Job drawing, mm, ordinate dimensions from the low corner. One solid piece. A direction names the side the tool comes from. Coordinates: 2 decimals unless noted, no trailing zeros. Loops run counter-clockwise (first coordinate to the right, second up) from the corner with the lowest first, then second, coordinate; pieces in that order, holes last. Notation, with made-up numbers: (53, 86) -> (107, 86) arc R17 cw to (107, 114) -> close; hole circle Ø3 at (-40, 22). An arc over 180 degrees is marked (long way). Use one line per item in the form item = value. Start each with the question number.
(1) Drill centre lines: L1, parallel to Y at x = 42, z = 11; L2, parallel to X at y = 54.5, z = 14.5. Where is each one in solid material? Low to high. Write a range as [from, to].
(2) Band-saw the part on C-C on z = 8.75. Give the cut face in (x, y).
(3) 3-axis set-ups, long thin cutter, end or side, ignore diameter. For the marked faces 1 and 2: which of +Z, -Z, +X, -X, +Y, -Y reach the whole face in a straight line?
(4) Pin check, flat tip, straight feed: P1, Ø4, axis at y = 35, z = 13, coming from the -X side. Stop position of the tip, or through.
(5) Band-saw the part on B-B on x = 105. Give the cut face in (y, z), then the cut area to 3 significant figures.
(6) Band-saw the part on A-A on y = 49.5. Give the cut face in (x, z).
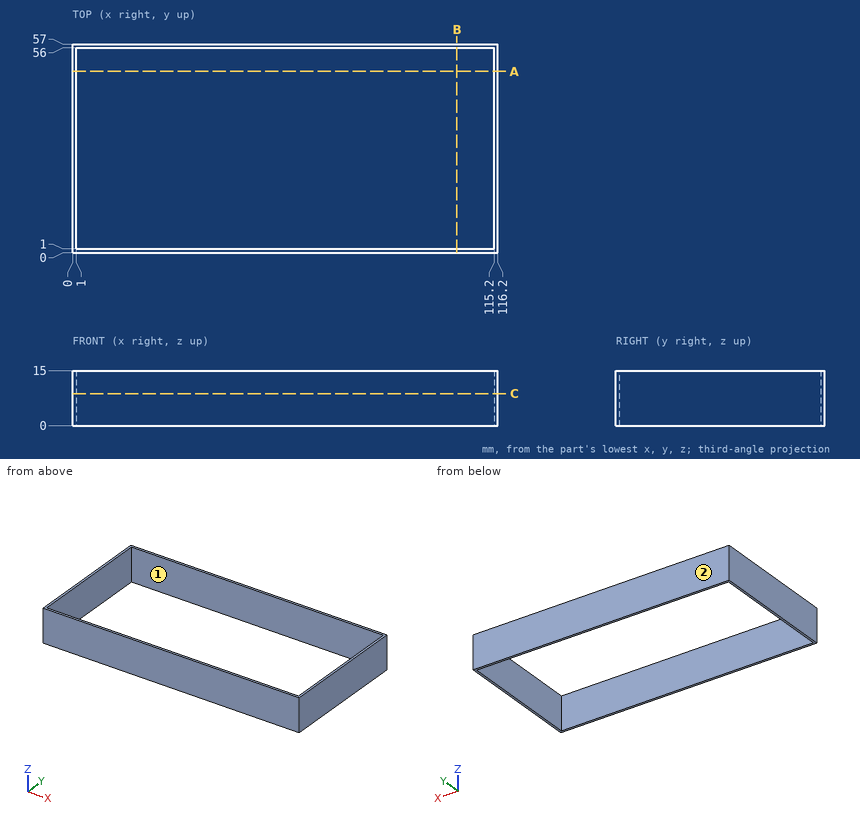
A:
q1.L1 = [0, 1], [56, 57]
q1.L2 = [0, 1], [115.2, 116.2]
q2.outline = (0, 0) -> (116.2, 0) -> (116.2, 57) -> (0, 57) -> close; hole (1, 1) -> (115.2, 1) -> (115.2, 56) -> (1, 56) -> close
q3.face_1 = +Z, -Z
q3.face_2 = +Z, -Z, +X, -X, +Y
q4.P1 = 0
q5.outline = (0, 0) -> (1, 0) -> (1, 15) -> (0, 15) -> close; (56, 0) -> (57, 0) -> (57, 15) -> (56, 15) -> close
q5.area = 30.0 mm²
q6.outline = (0, 0) -> (1, 0) -> (1, 15) -> (0, 15) -> close; (115.2, 0) -> (116.2, 0) -> (116.2, 15) -> (115.2, 15) -> close
